Verification items for the finished model (mm, model axes). A direction names the side the tool comes from. Give positions to 0.01 mm unless a question says otherwise; leave off trailing zeros. Order: outer loops, then holes, each group sorted by start corner. A loop starts at its lowest first (then second) coordinate and runs counter-clockwise, first axis right, second up.
(1) Sectioned sample at C-C on z = 1094.5. Record the cut outline in (x, y).
(2) Sectioned sample at B-B on y = -133. Record the cut outline in (x, z), plus the area to 3 significant figures.
(3) Sectioned sample at A-A on x = -41. Record the cut outline in (y, z).
(4) Mould release check, pull along Z, two halves, no side actions. Record for faces 1 (the face through (-173, -500, 986)), 2 (the face through (-181, -247, 16)), 3 (the face through (-173, -246, 2000)): pulls with the +Z half, pulls with the -Z half, needs draft (parallel to the pull), parting line crosses it, or undercut.
(5) Scan lines: L1, parallel to Y at x = -154.5, z = 1752.5; L2, parallel to Z at x = -316, y = -200; L3, parallel to X at y = -122.5, z = 643. Record each from-to range of solid material in increasing order.
(6) Gauge pin test, flat end, axial feed: pin 1 (3 mm diameter, centred on y = -448, z = 719.5, fed in from -X). Record the tip position at first contact, or that the pin passes through.
(7) Access from +Z, -Z, +X, -X, +Y, -Y to the whole of each face (thin tool, end or side, straight path). Record for faces 4 (the face through (-181, -16, 986)), 5 (the face through (-173, 0, 986)).
```python
from build123d import *

# Parameters (mm, degrees)
F0_W     = 45.8271801472
F0_H     = 53.0440360308
F1_DEPTH = 350
F2_DEPTH = 500
F3_DEPTH = 2000
F4_T     = -16


with BuildPart() as f1:
    # F0 (on Right) → F1 (new body)
    with BuildSketch(Plane.YZ):
        with Locations((-22.9135900736, 26.5220180154)):
            Rectangle(F0_W, F0_H)
    extrude(amount=-F1_DEPTH)

    # F2 (add): a face of the model
    f2_faces = [f1.faces().sort_by_distance(p)[0] for p in [
        (-175, 0, 26.5220180154),
    ]]
    extrude(f2_faces, amount=-F2_DEPTH)

    # F3 (add): a face of the model
    f3_faces = [f1.faces().sort_by_distance(p)[0] for p in [
        (-175, -250, 0),
    ]]
    extrude(f3_faces, amount=-F3_DEPTH)

    # F4
    f4_openings = [f1.faces().sort_by_distance(p)[0] for p in [
        (-350, -250, 1000),
    ]]
    offset(amount=F4_T, openings=f4_openings)


solid = f1.part
```
Ans:
1. outline: (-350, -500) - (0, -500) - (0, 0) - (-350, 0) - (-350, -16) - (-16, -16) - (-16, -484) - (-350, -484) - close
2. outline: (-350, 0) - (0, 0) - (0, 2000) - (-350, 2000) - (-350, 1984) - (-16, 1984) - (-16, 16) - (-350, 16) - close
2. area: 42,700 mm2
3. outline: (-500, 0) - (0, 0) - (0, 2000) - (-500, 2000) - close; hole (-484, 16) - (-16, 16) - (-16, 1984) - (-484, 1984) - close
4. face 1: needs draft
4. face 2: undercut
4. face 3: pulls with the +Z half
5. L1: y = -500 to -484, -16 to 0
5. L2: z = 0 to 16, 1984 to 2000
5. L3: x = -16 to 0
6. pin 1: stops at x = -16
7. face 4: -X
7. face 5: +Z, -Z, +X, -X, +Y
